Here's how the part is built. I have some questions about the finished solid (model axes, mm). Face numbers are marked on the shaded views. A direction names the side the tool comes from. Round coordinates to 2 decimals unless told otherwise and drop trailing zeros. Loops run counter-clockwise (first coordinate to the right, second up) from the corner with the lowest first, then second, coordinate; pieces in that order, holes last. Notation, with made-up numbers: M 88.5,11 L 138.5,11 A9 ccw 138.5,22 Z; hole C 40.5,48.5 d1. An arc over 180 degrees is marked long. Use a Markdown table: item, result.
from build123d import *

# Parameters (mm, degrees)
SKETCH_1_W          = 30
SKETCH_1_H          = 30
EXTRUDE_1_DEPTH     = 10
SKETCH_3_W          = 30
SKETCH_3_H          = 7
SKETCH_3_H_2        = 1.5
EXTRUDE_3_DEPTH     = 30
SKETCH_4_R          = 1.55
CUT_EXTRUDE_1_DEPTH = 30
SKETCH_5_R          = 3.5
SKETCH_5_R_2        = 1.55
CUT_EXTRUDE_2_DEPTH = 3


with BuildPart() as part:
    # 草图1 → 凸台-拉伸1 (new body)
    with BuildSketch(Plane(origin=(0, 0, 0), x_dir=(1, 0, 0), z_dir=(0, 1, 0))):
        Rectangle(SKETCH_1_W, SKETCH_1_H)
    extrude(amount=EXTRUDE_1_DEPTH)

    # 草图3 → 凸台-拉伸3 (add)
    with BuildSketch(Plane.XZ):
        with Locations((0, 10)):
            Rectangle(SKETCH_3_W, SKETCH_3_H)
        with Locations((0, 14.25)):
            Rectangle(SKETCH_3_W, SKETCH_3_H_2)
    extrude(amount=EXTRUDE_3_DEPTH)

    # 草图4 → 切除-拉伸1 (cut)
    with BuildSketch(Plane.XZ):
        with Locations(Location((5, 1, 0), (0, 0, 270))):
            Circle(SKETCH_4_R)
        with Locations(Location((5, -9, 0), (0, 0, 270))):
            Circle(SKETCH_4_R)
        with Locations(Location((-5, 1, 0), (0, 0, 270))):
            Circle(SKETCH_4_R)
        with Locations(Location((-5, -9, 0), (0, 0, 270))):
            Circle(SKETCH_4_R)
    extrude(amount=-CUT_EXTRUDE_1_DEPTH, mode=Mode.SUBTRACT)

    # 草图5 → 切除-拉伸2 (cut)
    # profile 1 of 4: a face of its own
    with BuildSketch(Plane.XZ):
        with Locations(Location((5, 1, 0), (0, 0, 270))):
            Circle(SKETCH_5_R)
        with Locations(Location((5, 1, 0), (0, 0, 270))):
            Circle(SKETCH_5_R_2, mode=Mode.SUBTRACT)
    # profile 2 of 4: a face of its own
    with BuildSketch(Plane.XZ):
        with Locations(Location((5, -9, 0), (0, 0, 270))):
            Circle(SKETCH_5_R)
        with Locations(Location((5, -9, 0), (0, 0, 270))):
            Circle(SKETCH_5_R_2, mode=Mode.SUBTRACT)
    # profile 3 of 4: a face of its own
    with BuildSketch(Plane.XZ):
        with Locations(Location((-5, -9, 0), (0, 0, 270))):
            Circle(SKETCH_5_R)
        with Locations(Location((-5, -9, 0), (0, 0, 270))):
            Circle(SKETCH_5_R_2, mode=Mode.SUBTRACT)
    # profile 4 of 4: a face of its own
    with BuildSketch(Plane.XZ):
        with Locations(Location((-5, 1, 0), (0, 0, 270))):
            Circle(SKETCH_5_R)
    extrude(amount=-CUT_EXTRUDE_2_DEPTH, mode=Mode.SUBTRACT)


solid = part.part
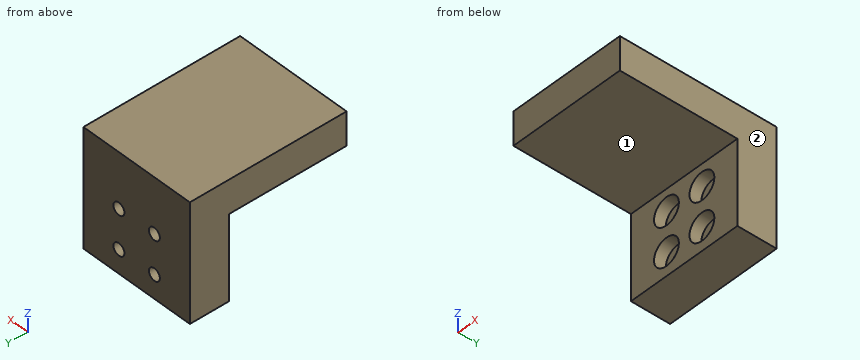
1. I need wall thicknesses on probe 1 along X at (y, z) = (6.5, -9); probe 2 along X at (y, z) = (1, -9); probe 3 along Y at (x, z) = (5.25, -2). Which ranges of each line are inside material? Lowest first, please. Write a range as from..to.
Answer sheet:
| item | result |
|---|---|
| probe 1 | -15..-6.55, -3.45..3.45, 6.55..15 |
| probe 2 | -15..-8.5, -1.5..1.5, 8.5..15 |
| probe 3 | 3..10 |
2. Imagine slicing it at D-D, the plane x = 12.5. Write out the boundary of the cut face in (y, z), then the cut area to 3 significant figures.
Answer sheet:
| item | result |
|---|---|
| outline | M -30,6.5 L 0,6.5 L 0,-15 L 10,-15 L 10,15 L -30,15 Z |
| area | 555 mm2 |
3. Imagine slicing it at B-B, the plane x = 5. Write out the boundary of the cut face in (y, z), then the cut area to 3 significant figures.
Answer sheet:
| item | result |
|---|---|
| outline | M -30,6.5 L 0,6.5 L 0,4.5 L 3,4.5 L 3,2.55 L 10,2.55 L 10,15 L -30,15 Z; M 0,-15 L 10,-15 L 10,-10.55 L 3,-10.55 L 3,-12.5 L 0,-12.5 Z; M 0,-5.5 L 3,-5.5 L 3,-7.45 L 10,-7.45 L 10,-0.55 L 3,-0.55 L 3,-2.5 L 0,-2.5 Z |
| area | 470 mm2 |
4. Imagine slicing it at C-C, the plane y = 7. Write out the boundary of the cut face in (x, z), then the cut area to 3 significant figures.
Answer sheet:
| item | result |
|---|---|
| outline | M -15,-15 L 15,-15 L 15,15 L -15,15 Z; hole C -5,-9 d3.1; hole C -5,1 d3.1; hole C 5,-9 d3.1; hole C 5,1 d3.1 |
| area | 870 mm2 |
5. Which directions (+Z, -Z, +X, -X, +Y, -Y) give clear straight access to the entire face, cutting with the end or side of a thin tool? Please do the marked faces 1 and 2.
Answer sheet:
| item | result |
|---|---|
| face 1 | -Z, +X, -X, -Y |
| face 2 | +Z, -Z, +X, +Y, -Y |
6. Imagine slicing it at A-A, the plane z = -9. Write out the boundary of the cut face in (x, y), then the cut area to 3 significant figures.
Answer sheet:
| item | result |
|---|---|
| outline | M -15,0 L -8.5,0 L -8.5,3 L -6.55,3 L -6.55,10 L -15,10 Z; M -3.45,3 L -1.5,3 L -1.5,0 L 1.5,0 L 1.5,3 L 3.45,3 L 3.45,10 L -3.45,10 Z; M 6.55,3 L 8.5,3 L 8.5,0 L 15,0 L 15,10 L 6.55,10 Z |
| area | 215 mm2 |
7. For pin 1 Ø7.5 at (x, z) = (3.5, 1.5) entering from -Y; pin 2 Ø5.5 at (x, z) = (5, -9) entering from -Y; pin 3 Ø6.5 at (x, z) = (-5, 1) entering from +Y; pin 4 Ø12 at (x, y) = (-5.5, -17.5) entering from -Z, each with a flat end and sliding along its axis, tell me the tip position at first contact or that it passes through.
Answer sheet:
| item | result |
|---|---|
| pin 1 | y = 0 |
| pin 2 | y = 3 |
| pin 3 | y = 10 |
| pin 4 | z = 6.5 |
